For this review, take the finished solid that the model builds, in its own axes (mm). Face numbers are marked on the shaded views. A direction names the side the tool comes from. Round coordinates to 2 decimals unless told otherwise and drop trailing zeros. Order: outer loops, then holes, each group sorted by start corner. A loop starts at its lowest first (then second) coordinate and runs counter-clockwise, first axis right, second up. Notation, with made-up numbers: (87.25, 82.5) -> (142.25, 82.5) arc R30 ccw to (142.25, 120.5) -> close; hole circle Ø9 at (55.5, 35.5). An arc over 180 degrees is marked (long way). Answer in a Markdown table with one row per item.
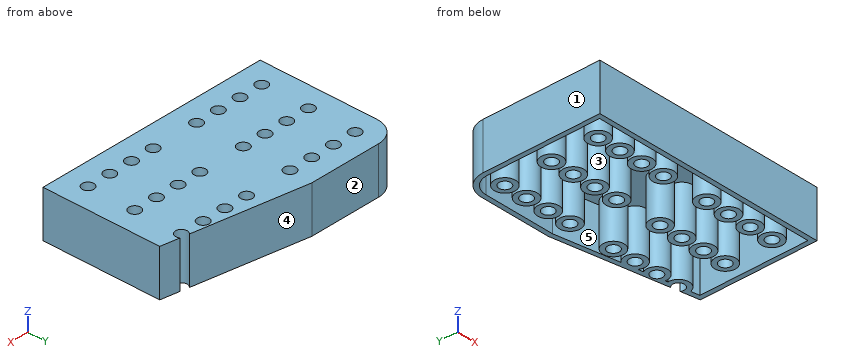
```python
from build123d import *

# Parameters (mm, degrees)
F1_DEPTH = 25.4
F2_R     = 3.175
F3_DEPTH = 25.4
F4_T     = -2.54


# Not quite as in the source:
# - a shell that OpenCascade refuses in one call is made with other operations: the cavity is built on its own and cut out


with BuildPart() as f1:
    # F0 (on Top) → F1 (new body)
    with BuildSketch(Plane.XY):
        with BuildLine():
            Line((51.71799147, 0), (12.7, 0))
            ThreePointArc((12.7, 0), (3.7197438789, -3.7197438789), (0, -12.7))
            Line((0, -12.7), (0, -76.2))
            Line((0, -76.2), (127, -76.2))
            Line((127, -76.2), (127, -12.7))
            Line((127, -12.7), (51.71799147, 0))
        make_face()
    extrude(amount=F1_DEPTH)

    # F2 (on face) → F3 (cut)
    with BuildSketch(Plane.XY.offset(25.4)):
        with Locations((12.7, -12.7)):
            Circle(F2_R)
        with Locations((12.7, -38.1)):
            Circle(F2_R)
        with Locations((12.7, -63.5)):
            Circle(F2_R)
        with Locations((25.4, -12.7)):
            Circle(F2_R)
        with Locations((25.4, -38.1)):
            Circle(F2_R)
        with Locations((25.4, -63.5)):
            Circle(F2_R)
        with Locations((38.1, -12.7)):
            Circle(F2_R)
        with Locations((38.1, -38.1)):
            Circle(F2_R)
        with Locations((38.1, -63.5)):
            Circle(F2_R)
        with Locations((50.8, -12.7)):
            Circle(F2_R)
        with Locations((50.8, -38.1)):
            Circle(F2_R)
        with Locations((50.8, -63.5)):
            Circle(F2_R)
        with Locations((114.3, -12.7)):
            Circle(F2_R)
        with Locations((101.6, -12.7)):
            Circle(F2_R)
        with Locations((88.9, -12.7)):
            Circle(F2_R)
        with Locations((114.3, -38.1)):
            Circle(F2_R)
        with Locations((101.6, -38.1)):
            Circle(F2_R)
        with Locations((88.9, -38.1)):
            Circle(F2_R)
        with Locations((114.3, -63.5)):
            Circle(F2_R)
        with Locations((101.6, -63.5)):
            Circle(F2_R)
        with Locations((88.9, -63.5)):
            Circle(F2_R)
        with Locations((76.2, -63.5)):
            Circle(F2_R)
        with Locations((76.2, -38.1)):
            Circle(F2_R)
        with Locations((76.2, -12.7)):
            Circle(F2_R)
    extrude(amount=-F3_DEPTH, mode=Mode.SUBTRACT)

    # F4: a shell. OpenCascade refuses it in one call, so the cavity is built on its own and cut out:
    # the body offset inwards by the wall thickness, plus a prism from it out through each open face.
    f4_core = offset(f1.part, amount=F4_T, kind=Kind.INTERSECTION, mode=Mode.PRIVATE)
    f4_exits = [f4_core.faces().sort_by_distance(p)[0] for p in [
        (61.661975, -40.163324, 2.54),
    ]]
    add(f4_core, mode=Mode.SUBTRACT)
    extrude(f4_exits, amount=-F4_T, mode=Mode.SUBTRACT)


solid = f1.part
```
Q1. Take a section at C-C, the plane x = 114.3. Write out the cut boundary in (y, z) (3 decimals), then the cut area to 3 significant figures.
Answer key:
| item | result |
|---|---|
| outline | (-76.2, 0) -> (-73.66, 0) -> (-73.66, 22.86) -> (-69.215, 22.86) -> (-69.215, 0) -> (-66.675, 0) -> (-66.675, 25.4) -> (-76.2, 25.4) -> close; (-60.325, 0) -> (-57.785, 0) -> (-57.785, 22.86) -> (-43.815, 22.86) -> (-43.815, 0) -> (-41.275, 0) -> (-41.275, 25.4) -> (-60.325, 25.4) -> close; (-34.925, 0) -> (-32.385, 0) -> (-32.385, 22.86) -> (-18.415, 22.86) -> (-18.415, 0) -> (-15.875, 0) -> (-15.875, 25.4) -> (-34.925, 25.4) -> close |
| area | 469 mm^2 |
Q2. Tool access review of the marked faces 4 and 5: name each direction out of +Z, -Z, +X, -X, +Y, -Y from which nothing blocks a thin tool from reaching the whole face with its end or side.
Answer key:
| item | result |
|---|---|
| face 4 | +Z, -Z, +X, +Y |
| face 5 | -Z |
Q3. Clearance check with flat-ended pins moving along their axes: pin 1 Ø4 at (x, z) = (62, 8.5) entering from +Y; pin 2 Ø6 at (x, y) = (65, -62.5) entering from -Z. State where each tip first meets the part, or that it passes through.
Answer key:
| item | result |
|---|---|
| pin 1 | stops at y = -1.4 |
| pin 2 | stops at z = 22.86 |
Q4. Take a section at D-D, the plane y = -20. Write out the cut boundary in (x, z).
Answer key:
| item | result |
|---|---|
| outline | (0, 0) -> (2.54, 0) -> (2.54, 22.86) -> (124.46, 22.86) -> (124.46, 0) -> (127, 0) -> (127, 25.4) -> (0, 25.4) -> close |
Q5. To check wall thickness, follow probe 1 along Y at (x, z) = (114.3, 13.5) (3 decimals); probe 2 along X at (y, z) = (-26, 21); probe 3 along Y at (x, z) = (111, 11.75). State the ranges of each line that lie inside material, in increasing order.
Answer key:
| item | result |
|---|---|
| probe 1 | y = -76.2 to -73.66, -69.215 to -66.675, -60.325 to -57.785, -43.815 to -41.275, -34.925 to -32.385, -18.415 to -15.875 |
| probe 2 | x = 0 to 2.54, 124.46 to 127 |
| probe 3 | y = -76.2 to -73.66, -68.17 to -58.83, -42.77 to -33.43, -17.37 to -10 |
Q6. The part is to be moulded in two halves that separate along X. For the marked faces 1, 2 and 3, say which applies: +X half, -X half, draft (parallel to the pull), parting line (faces both ways), or undercut.
Answer key:
| item | result |
|---|---|
| face 1 | -X half |
| face 2 | draft |
| face 3 | undercut |
Q7. Take a section at A-A, the plane x = 25.4. Give the number of separate pieces and of enclosed holes in the cut face, then the cut area to 3 significant figures.
Answer key:
| item | result |
|---|---|
| separate pieces | 4 |
| enclosed holes | 0 |
| area | 610 mm^2 |
